Answer from the drawing. Dimensions are ordinates in mm from the lowest x, y and z of the part. A direction names the side the tool comes from. Coordinates: 2 decimals unless noted, no trailing zeros. Write each loop counter-clockwise with the first axis right and the second up, starting at its lowest first coordinate (ties: lowest second). Pieces come first, ordered by that corner, then holes. Notation, with made-up numbers: (75.25, 14) - (134.25, 14) arc R9 ccw to (134.25, 25) - close; hole circle Ø11 at (14.25, 84.5). An arc over 180 degrees is marked (long way). Return JSON: item names as keys, results as strings.
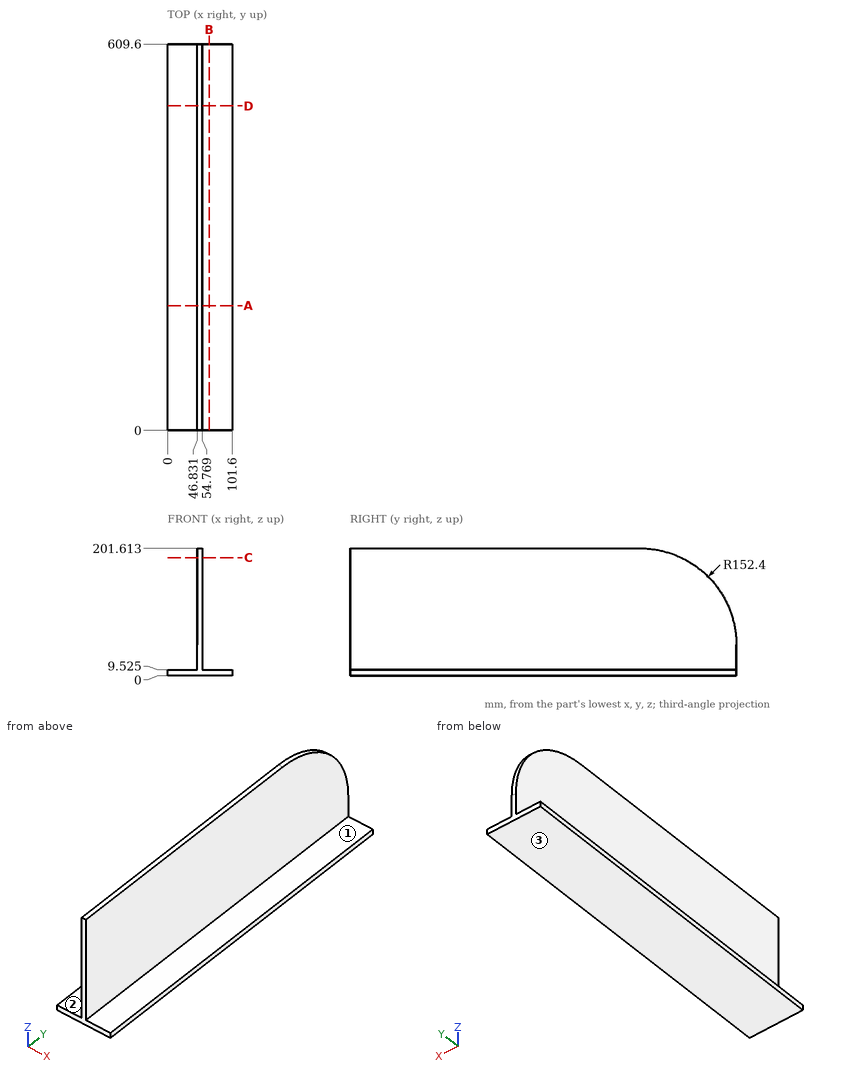
(1) Straight lines are drawn through the part: line 1 (Z direction, x = 61, y = 338) (1 decimal); line 2 (X direction, y = 211, z = 70.5); line 3 (Z direction, x = 51.5, y = 495). For each, find the intervals that lie inside material, in ascending order. Write a range as from..to.
Answer:
{"line 1": "0..9.5", "line 2": "46.83..54.77", "line 3": "0..196.85"}
(2) A cutting plane is placed at A-A (y = 196.5). Determine the outline of the cut face in (x, z) (1 decimal).
Answer:
{"outline": "(0, 0) - (101.6, 0) - (101.6, 9.5) - (54.8, 9.5) - (54.8, 201.6) - (46.8, 201.6) - (46.8, 9.5) - (0, 9.5) - close"}
(3) A cutting plane is placed at D-D (y = 512). Determine the outline of the cut face in (x, z) (1 decimal), and give its area (3 significant figures).
Answer:
{"outline": "(0, 0) - (101.6, 0) - (101.6, 9.5) - (54.8, 9.5) - (54.8, 191.4) - (46.8, 191.4) - (46.8, 9.5) - (0, 9.5) - close", "area": "2,410 mm²"}
(4) A cutting plane is placed at C-C (z = 187). Determine the outline of the cut face in (x, y).
Answer:
{"outline": "(46.83, 0) - (54.77, 0) - (54.77, 522.32) - (46.83, 522.32) - close"}
(5) Flat-ended cylindrical pins translate along their axes: P1, Ø4, axis at x = 30.5, y = 101, coming from the +Z side (1 decimal); P2, Ø2, axis at y = 441.5, z = 60.5, coming from the -X side. Find the tip coordinate at first contact, or state that the pin passes through.
Answer:
{"P1": "z = 9.5", "P2": "x = 46.83"}
(6) Which of the six approach directions +Z, -Z, +X, -X, +Y, -Y give full straight-line access (tool end or side, diameter ignored) to the marked faces 1, 2 and 3?
Answer:
{"face 1": "+Z, +X, +Y, -Y", "face 2": "+Z, -X, +Y, -Y", "face 3": "-Z, +X, -X, +Y, -Y"}
(7) A cutting plane is placed at B-B (x = 65.5). Determine the outline of the cut face in (y, z) (1 decimal), and give its area (3 significant figures).
Answer:
{"outline": "(0, 0) - (609.6, 0) - (609.6, 9.5) - (0, 9.5) - close", "area": "5,810 mm²"}
